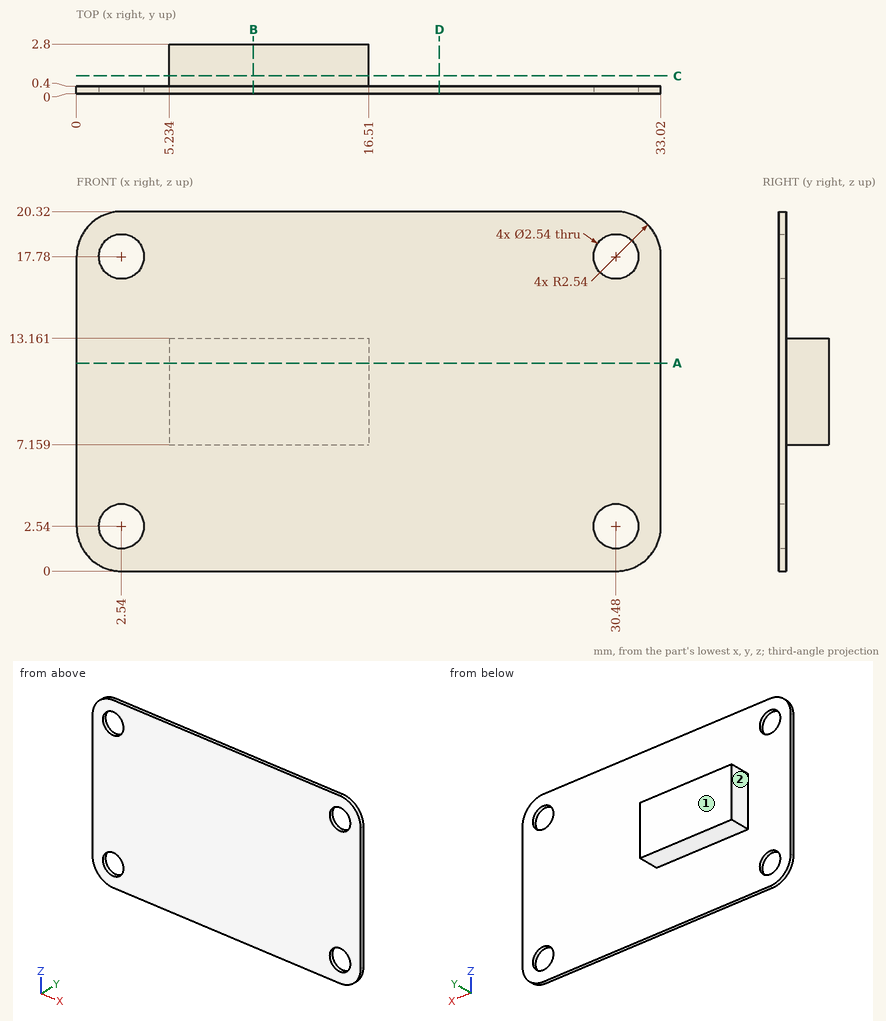
Study the drawing (mm; zero at the part's minimum x, y, z) and answer. A direction names the side the tool comes from. Coordinates: 2 decimals unless noted, no trailing zeros. Loops run counter-clockwise (first coordinate to the right, second up) from the corner with the lowest first, then second, coordinate; pieces in that order, holes last. Notation, with made-up numbers: M -40,-19.5 L -29,-19.5 A31 ccw -29,7.5 Z; hole C 41,-21.75 d2. An arc over 180 degrees is marked long. Answer in a Markdown table with one row per item.
1) Find section D-D (x = 20.5). Determine the outline of the cut face in (y, z).
Answers below:
| item | result |
|---|---|
| outline | M 0,0 L 0.4,0 L 0.4,20.32 L 0,20.32 Z |
2) Find section C-C (y = 1). Determine the outline of the cut face in (x, z), then the cut area to 3 significant figures.
Answers below:
| item | result |
|---|---|
| outline | M 5.23,7.16 L 16.51,7.16 L 16.51,13.16 L 5.23,13.16 Z |
| area | 67.7 mm^2 |
3) Which of the six approach directions +Z, -Z, +X, -X, +Y, -Y give full straight-line access (tool end or side, diameter ignored) to the marked faces 1 and 2?
Answers below:
| item | result |
|---|---|
| face 1 | +Z, -Z, +X, -X, +Y |
| face 2 | +Z, -Z, -X, +Y |
4) Find the intervals of material crossed by probe 1 along X at (y, z) = (0.15, 17.78); probe 2 along Y at (x, z) = (15.5, 16.25); probe 3 along Z at (x, y) = (12, 0.65), in increasing order.
Answers below:
| item | result |
|---|---|
| probe 1 | 0 to 1.27, 3.81 to 29.21, 31.75 to 33.02 |
| probe 2 | 0 to 0.4 |
| probe 3 | 7.16 to 13.16 |
5) Given pin 1 (5 mm diameter, centred on x = 22.5, z = 9.5, fed in from +Y); pin 2 (1.5 mm diameter, centred on x = 29, y = 1.5, fed in from -Z); pin 3 (0.7 mm diameter, centred on y = 1.5, z = 11.5, fed in from +X), each flat-ended and moving along its own axis, determine where each tip first touches the part or whether it passes through.
Answers below:
| item | result |
|---|---|
| pin 1 | y = 0.4 |
| pin 2 | through |
| pin 3 | x = 16.51 |
6) Find section A-A (z = 11.75). Determine the outline of the cut face in (x, y).
Answers below:
| item | result |
|---|---|
| outline | M 0,0 L 33.02,0 L 33.02,0.4 L 16.51,0.4 L 16.51,2.8 L 5.23,2.8 L 5.23,0.4 L 0,0.4 Z |
7) Find section B-B (x = 10). Determine the outline of the cut face in (y, z).
Answers below:
| item | result |
|---|---|
| outline | M 0,0 L 0.4,0 L 0.4,7.16 L 2.8,7.16 L 2.8,13.16 L 0.4,13.16 L 0.4,20.32 L 0,20.32 Z |
